Build history of the part. All positions in model axes, mm. A direction names the side the tool comes from. Round coordinates to 2 decimals unless told otherwise and drop trailing zeros. Write each loop counter-clockwise with the first axis right and the second up, starting at its lowest first coordinate (ties: lowest second). Pieces come first, ordered by that corner, then holes. Notation, with made-up numbers: M 21,34 L 47,34 A23 ccw 47,57 Z; hole C 83.5,87.25 d4. An arc over 180 degrees is marked long. Use a Markdown table: item, result.
from build123d import *

# Parameters (mm, degrees)
SKETCH1_W               = 19.800000024
SKETCH1_H               = 125.800000114
SKETCH1_R               = 3.3
SKETCH1_W_2             = 19.05
BOSS_EXTRUDE1_DEPTH     = 3.175
CUT_EXTRUDE1_DEPTH      = 70.315172458
CUT_EXTRUDE1_DEPTH_BACK = 70.315172458
FILLET1_R               = 3.175
SKETCH7_W               = 2.54
SKETCH7_H               = 125.800000114
EXTRUDE_THIN1_DEPTH     = 15.525155132
FILLET2_R               = 3.175


with BuildPart() as part:
    # Sketch1 → Boss-Extrude1 (new body)
    # profile 1 of 2: a face of its own
    with BuildSketch(Plane.XY):
        Rectangle(SKETCH1_W, SKETCH1_H)
        with Locations((0, -53.000000045)):
            Circle(SKETCH1_R, mode=Mode.SUBTRACT)
        with Locations((0, 53.000000045)):
            Circle(SKETCH1_R, mode=Mode.SUBTRACT)
    # profile 2 of 2: a face of its own
    with BuildSketch(Plane.XY):
        with Locations((-19.425000012, 0)):
            Rectangle(SKETCH1_W_2, SKETCH1_H)
    extrude(amount=BOSS_EXTRUDE1_DEPTH)

    # Sketch6 → Cut-Extrude1 (cut, two sides: drawn at the far end of the back side and taken through both)
    with BuildSketch(Plane.XY.offset(3.175).offset(-CUT_EXTRUDE1_DEPTH_BACK)):
        with BuildLine():
            Line((4.7625, 38.337500033), (4.7625, 12.462499967))
            ThreePointArc((4.7625, 12.462499967), (0, 7.699999967), (-4.7625, 12.462499967))
            Line((-4.7625, 12.462499967), (-4.7625, 38.337500033))
            ThreePointArc((-4.7625, 38.337500033), (0, 43.100000033), (4.7625, 38.337500033))
        make_face()
        with BuildLine():
            Line((4.7625, -12.462499967), (4.7625, -38.337500033))
            ThreePointArc((4.7625, -38.337500033), (0, -43.100000033), (-4.7625, -38.337500033))
            Line((-4.7625, -38.337500033), (-4.7625, -12.462499967))
            ThreePointArc((-4.7625, -12.462499967), (0, -7.699999967), (4.7625, -12.462499967))
        make_face()
    extrude(amount=CUT_EXTRUDE1_DEPTH + CUT_EXTRUDE1_DEPTH_BACK, mode=Mode.SUBTRACT)

    # Fillet1
    fillet1_edges = [part.edges().sort_by_distance(p)[0] for p in [
        (9.900000012, 62.900000057, 1.5875),
        (9.900000012, -62.900000057, 1.5875),
    ]]
    fillet(fillet1_edges, radius=FILLET1_R)

    # Sketch7 → Extrude-Thin1 (add)
    with BuildSketch(Plane.XY.offset(3.175)):
        with Locations((-27.680000012, 0)):
            Rectangle(SKETCH7_W, SKETCH7_H)
    extrude(amount=EXTRUDE_THIN1_DEPTH)

    # Fillet2
    fillet2_edges = [part.edges().sort_by_distance(p)[0] for p in [
        (-27.680000012, -62.900000057, 18.700155132),
        (-27.680000012, 62.900000057, 18.700155132),
        (-26.410000012, 0, 3.175),
        (-28.950000012, 0, 0),
    ]]
    fillet(fillet2_edges, radius=FILLET2_R)


solid = part.part
Q1. Cut at C-C on z = 1.5. Count the separate pieces of the cut face and the enclosed holes in it, and give its area (3 significant figures).
Response values:
| item | result |
|---|---|
| separate pieces | 1 |
| enclosed holes | 4 |
| area | 4,120 mm2 |
Q2. Cut at A-A on x = 0. Give the cut face in (y, z) (3 decimals).
Response values:
| item | result |
|---|---|
| outline | M -62.9,0 L -56.3,0 L -56.3,3.175 L -62.9,3.175 Z; M -49.7,0 L -43.1,0 L -43.1,3.175 L -49.7,3.175 Z; M -7.7,0 L 7.7,0 L 7.7,3.175 L -7.7,3.175 Z; M 43.1,0 L 49.7,0 L 49.7,3.175 L 43.1,3.175 Z; M 56.3,0 L 62.9,0 L 62.9,3.175 L 56.3,3.175 Z |
Q3. Drill centre lines: L1, parallel to Y at x = 0, z = 1.95; L2, parallel to Z at x = 6, y = 29 (3 decimals); L3, parallel to X at y = -53, z = 1.35. Where is each one in solid material? Low to high.
Response values:
| item | result |
|---|---|
| L1 | y = -62.9 to -56.3, -49.7 to -43.1, -7.7 to 7.7, 43.1 to 49.7, 56.3 to 62.9 |
| L2 | z = 0 to 3.175 |
| L3 | x = -28.37 to -3.3, 3.3 to 9.9 |
Q4. Cut at D-D on y = -46. Give the cut face in (x, z) (3 decimals).
Response values:
| item | result |
|---|---|
| outline | M -28.95,3.175 A3.175 ccw -25.775,0 L 9.9,0 L 9.9,3.175 L -23.235,3.175 A3.175 cw -26.41,6.35 L -26.41,18.7 L -28.95,18.7 Z |
Q5. Which spindle directions (+Z, -Z, +X, -X, +Y, -Y) get a long thin tool onto all of the face, cutting with end or side? Do faces 5 (the flat face through (-15, 62.9, 3)), 6 (the flat face through (-26.41, -1, 12)), 7 (the flat face through (-4.762, 25, 2)). Say none if no direction does.
Response values:
| item | result |
|---|---|
| face 5 | +Z, -Z, +X, -X, +Y |
| face 6 | +Z, +X, +Y, -Y |
| face 7 | +Z, -Z |
Q6. Cut at B-B on y = 53. Give the cut face in (x, z) (3 decimals), and give its area (3 significant figures).
Response values:
| item | result |
|---|---|
| outline | M -28.95,3.175 A3.175 ccw -25.775,0 L -3.3,0 L -3.3,3.175 L -23.235,3.175 A3.175 cw -26.41,6.35 L -26.41,18.7 L -28.95,18.7 Z; M 3.3,0 L 9.9,0 L 9.9,3.175 L 3.3,3.175 Z |
| area | 142 mm2 |
Q7. Drop flat-ended pins along their axis: P1, Ø1, axis at y = 5, z = 5, coming from the +X side; P2, Ø5, axis at x = -19, y = 22.5, coming from the +Z side (3 decimals); P3, Ø1.6, axis at y = -31.5, z = 1.5, coming from the -X side. Give the stop position or say it passes through.
Response values:
| item | result |
|---|---|
| P1 | stops at x = -25.82 |
| P2 | stops at z = 3.175 |
| P3 | stops at x = -28.83 |
Q8. Two-plate mould, pull along Y, no slides. Class faces 1 (the cylindrical face through (0.1, 7.7, 1.6)), 2 (the flat face through (-4.762, -26, 2)), 3 (the cylindrical face through (8.95, -61.99, 1.61)), 4 (the flat face through (-7, 1, 3.175)): +Y half, -Y half, draft (parallel to the pull), parting line (faces both ways), or undercut.
Response values:
| item | result |
|---|---|
| face 1 | undercut |
| face 2 | undercut |
| face 3 | -Y half |
| face 4 | draft |
